The listing builds one solid part. Answer for the finished solid, in the listing's coordinates (mm). A direction names the side the tool comes from. Round coordinates to 2 decimals unless told otherwise and drop trailing zeros. Write each loop counter-clockwise with the first axis right and the second up, starting at its lowest first coordinate (ties: lowest second). Pieces come first, ordered by that corner, then holes. Notation, with made-up numbers: M -2,-22.75 L 12,-22.75 A30 cw 12,13.25 Z; hole C -32,-19 d1. An arc over 180 degrees is marked long. Write each question's results on one line, items separated by ' | '.
from build123d import *

# Parameters (mm, degrees)
BOSS_EXTRUDE1_DEPTH = 1.5875


with BuildPart() as part:
    # Sketch2 → Boss-Extrude1 (new body, symmetric)
    with BuildSketch(Plane.XY):
        Polygon((0, 0), (18, 0), (18, 11.675), (21.175, 11.675), (21.175, 20.675), (18, 20.675), (18, 32.35), (0, 32.35), (0, 20.675), (-3.175, 20.675), (-3.175, 11.675), (0, 11.675), align=None)
        Polygon((9, 29.35), (4.5, 29.35), (4.5, 26.175), (13.5, 26.175), (13.5, 29.35), align=None, mode=Mode.SUBTRACT)
        Polygon((13.5, 3), (9, 3), (4.5, 3), (4.5, 6.175), (13.5, 6.175), align=None, mode=Mode.SUBTRACT)
        Polygon((9, 8.675), (13, 8.675), (13, 18.675), (5, 18.675), (5, 8.675), align=None, mode=Mode.SUBTRACT)
    extrude(amount=BOSS_EXTRUDE1_DEPTH, both=True)


solid = part.part
1) Section B-B (z = -0.7) is taken. Determine the outline of the cut face in (x, y) (3 decimals), then the cut area to 3 significant figures.
Return value:
outline: M -3.175,11.675 L 0,11.675 L 0,0 L 18,0 L 18,11.675 L 21.175,11.675 L 21.175,20.675 L 18,20.675 L 18,32.35 L 0,32.35 L 0,20.675 L -3.175,20.675 Z; hole M 4.5,3 L 13.5,3 L 13.5,6.175 L 4.5,6.175 Z; hole M 4.5,26.175 L 13.5,26.175 L 13.5,29.35 L 4.5,29.35 Z; hole M 5,8.675 L 13,8.675 L 13,18.675 L 5,18.675 Z | area: 502 mm²
2) The mould has two halves that part along X. Classify faces 1 (the face through (9, 3, 0)), 2 (the face through (18, 26, 0)), 3 (the face through (9, 20, -1.588)): +X half, -X half, draft (parallel to the pull), parting line (faces both ways), or undercut.
Return value:
face 1: undercut | face 2: +X half | face 3: draft
3) Each of these flat-tipped pins is pushed along its axis until it touches: pin 1 (1.6 mm diameter, centred on y = 28.5, z = 0, fed in from +X); pin 2 (2 mm diameter, centred on x = 9.5, y = 10.5, fed in from +Z); pin 3 (1 mm diameter, centred on y = 3.5, z = -0.5, fed in from -X); pin 4 (1 mm diameter, centred on x = 19.5, z = 0, fed in from +Y) (3 decimals). Where does it stop, or does it pass through?
Return value:
pin 1: x = 18 | pin 2: through | pin 3: x = 0 | pin 4: y = 20.675
4) A tool of negligible diameter and unlimited length cuts with its end or side. For faces 4 (the face through (-3.175, 16, 0)), 5 (the face through (-2, 20.675, 0)), 6 (the face through (18, 6, 0)), 7 (the face through (9, 32.35, 0)), 8 (the face through (4.5, 5, 0)), from which of +Z, -Z, +X, -X, +Y, -Y can it reach the whole face along a straight path? Write none if from no direction.
Return value:
face 4: +Z, -Z, -X, +Y, -Y | face 5: +Z, -Z, -X, +Y | face 6: +Z, -Z, +X, -Y | face 7: +Z, -Z, +X, -X, +Y | face 8: +Z, -Z
5) Section A-A (x = 8) is taken. State how many separate pieces and enclosed holes the cut face has, then the cut area to 3 significant figures.
Return value:
separate pieces: 4 | enclosed holes: 0 | area: 50.8 mm²
6) Section D-D (y = 15) is taken. Determine the outline of the cut face in (x, z) (1 decimal).
Return value:
outline: M -3.2,-1.6 L 5,-1.6 L 5,1.6 L -3.2,1.6 Z; M 13,-1.6 L 21.2,-1.6 L 21.2,1.6 L 13,1.6 Z
7) Section C-C (y = 10.5) is taken. Determine the outline of the cut face in (x, z).
Return value:
outline: M 0,-1.59 L 5,-1.59 L 5,1.59 L 0,1.59 Z; M 13,-1.59 L 18,-1.59 L 18,1.59 L 13,1.59 Z
8) Find the intervals of material crossed by line 1 (Y direction, x = 9.25, z = 1.3) (3 decimals); line 2 (X direction, y = 28.5, z = -0.5); line 3 (X direction, y = 11, z = -0.05), in increasing order.
Return value:
line 1: 0 to 3, 6.175 to 8.675, 18.675 to 26.175, 29.35 to 32.35 | line 2: 0 to 4.5, 13.5 to 18 | line 3: 0 to 5, 13 to 18
